Geometry check sheet. Reference: the model listing, model coordinates, mm. Round coordinates to 2 decimals unless told otherwise and drop trailing zeros. Write each loop counter-clockwise with the first axis right and the second up, starting at its lowest first coordinate (ties: lowest second). Pieces come first, ordered by that corner, then holes. Notation, with made-up numbers: (-33.75, 84.5) - (24.25, 84.5) arc R12 cw to (24.25, 88.5) - close; hole circle Ø8 at (31, -20.5). An arc over 180 degrees is marked (long way). Return JSON: item names as keys, results as strings.
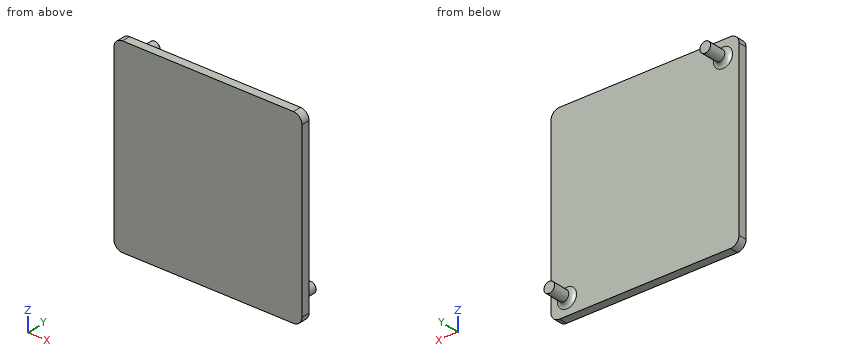
```python
from build123d import *

# Parameters (mm, degrees)
SKETCH1_W           = 44
SKETCH1_H           = 44
BOSS_EXTRUDE1_DEPTH = 2
SKETCH2_R           = 1.25
BOSS_EXTRUDE4_DEPTH = 5
FILLET4_R           = 2
FILLET5_R           = 1


with BuildPart() as part:
    # Sketch1 → Boss-Extrude1 (new body)
    with BuildSketch(Plane(origin=(0, 0, 0), x_dir=(1, 0, 0), z_dir=(0, 1, 0))):
        with Locations((22, 22)):
            Rectangle(SKETCH1_W, SKETCH1_H)
    extrude(amount=BOSS_EXTRUDE1_DEPTH)

    # Sketch2 → Boss-Extrude4 (add)
    with BuildSketch(Plane(origin=(0, 2, 0), x_dir=(1, 0, 0), z_dir=(0, 1, 0))):
        with Locations(Location((3.75, 3.75, 0), (0, 0, 90))):
            Circle(SKETCH2_R)
        with Locations(Location((40.25, 40.25, 0), (0, 0, 90))):
            Circle(SKETCH2_R)
    extrude(amount=BOSS_EXTRUDE4_DEPTH)

    # Fillet4
    fillet4_edges = [part.edges().sort_by_distance(p)[0] for p in [
        (0, 1, -44),
        (44, 1, -44),
        (44, 1, 0),
        (0, 1, 0),
    ]]
    fillet(fillet4_edges, radius=FILLET4_R)

    # Fillet5
    fillet5_edges = [part.edges().sort_by_distance(p)[0] for p in [
        (40.25, 2, -39),
        (3.75, 2, -2.5),
    ]]
    fillet(fillet5_edges, radius=FILLET5_R)


solid = part.part
```
(1) Gauge pin test, flat ends, axial feed: pin 1 (6 mm diameter, centred on x = 17.5, z = -26, fed in from +Y); pin 2 (4 mm diameter, centred on x = 5.5, y = 4.5, fed in from +Z). Record the tip position at first contact, or that the pin passes through.
Response values:
{"pin 1": "stops at y = 2", "pin 2": "stops at z = -2.5"}
(2) Section check A-A, the plane x = 3.75. Enter the section's corners in (y, z), plus the area to 3 significant figures.
Response values:
{"outline": "(0, -44) - (2, -44) - (2, -6) arc R1 cw to (3, -5) - (7, -5) - (7, -2.5) - (3, -2.5) arc R1 cw to (2, -1.5) - (2, 0) - (0, 0) - close", "area": "101 mm^2"}
(3) Section check B-B, the plane z = -3.75. Enter the section's corners in (x, y).
Response values:
{"outline": "(0, 0) - (44, 0) - (44, 2) - (6, 2) arc R1 cw to (5, 3) - (5, 7) - (2.5, 7) - (2.5, 3) arc R1 cw to (1.5, 2) - (0, 2) - close"}
(4) Section check D-D, the plane z = -26. Enter the section's corners in (x, y).
Response values:
{"outline": "(0, 0) - (44, 0) - (44, 2) - (0, 2) - close"}
(5) Material ranges on line 1 along Y through (x, z) = (27, -30); line 2 along Y through (x, z) = (42, -40.5); line 3 along X through (y, z) = (6, -39.5), recorded low to high. Write a range as [from, to].
Response values:
{"line 1": "y = [0, 2]", "line 2": "y = [0, 2.12]", "line 3": "x = [39.25, 41.25]"}
(6) Section check C-C, the plane y = 5. Enter the section's corners in (x, z).
Response values:
{"outline": "circle Ø2.5 at (3.75, -3.75); circle Ø2.5 at (40.25, -40.25)"}
